Autodesk Inventor part; units mm, degrees
ref_plane "end_2_XY" through (22.3, 10.5, 6.25) normal (0, 1, 0) x (1, 0, 0)
ref_plane "end_2_YZ" through (22.3, 10.5, 6.25) normal (1, 0, 0) x (0, 0, -1)
ref_plane "end_2_ZX" through (22.3, 10.5, 6.25) normal (0, 0, -1) x (0, 1, 0)
sketch "Sketch_77" plane through (0, 0, 0) normal (0, 0, 1) x (1, 0, 0)
  line L0 (0, 7.9) -> (0, -7.9)
  line L1 (0, -7.9) -> (16, -7.9)
  line L2 (16, -7.9) -> (16, 7.9)
  line L3 (16, 7.9) -> (0, 7.9)
  circle A0 centre (12, 0) radius 1.5
  circle A1 centre (4, 0) radius 1.5
extrude "Extrusion1" add sketch "Sketch_77" along normal blind 2
sketch "Sketch_78" plane through (0, 7.9, 0) normal (0, 1, 0) x (1, 0, 0)
  arc A0 (0, -4.5344) -> (0.6773, -5.4809) centre (1, -4.5344) ccw
  line L0 (0.6773, -5.4809) -> (20.283, -12.1656)
  arc A1 (20.283, -12.1656) -> (22.3, 0) centre (22.3, -6.25) ccw
  line L1 (22.3, 0) -> (0, 0)
  line L2 (0, 0) -> (0, -4.5344)
extrude "Extrusion2" add sketch "Sketch_78" along normal blind 1.85
sketch "Sketch_79" plane through (0, -7.9, 0) normal (0, 1, 0) x (1, 0, 0)
  arc A0 (0, -4.5344) -> (0.6773, -5.4809) centre (1, -4.5344) ccw
  line L0 (0.6773, -5.4809) -> (20.283, -12.1656)
  arc A1 (20.283, -12.1656) -> (22.3, 0) centre (22.3, -6.25) ccw
  line L1 (22.3, 0) -> (0, 0)
  line L2 (0, 0) -> (0, -4.5344)
extrude "Extrusion3" add sketch "Sketch_79" against normal blind 1.85
sketch "Sketch_80" plane through (0, 9.6, 0) normal (0, 1, 0) x (1, 0, 0)
  circle A0 centre (22.3, -6.25) radius 3
extrude "Extrusion4" add sketch "Sketch_80" along normal blind 1.4
sketch "Sketch_81" plane through (0, -9.6, 0) normal (0, 1, 0) x (1, 0, 0)
  circle A0 centre (22.3, -6.25) radius 3
extrude "Extrusion5" add sketch "Sketch_81" along normal mid plane 2.8
sketch "Sketch_82" plane through (0, 9.6, 0) normal (0, 1, 0) x (1, 0, 0)
  arc A0 (0, -4.5344) -> (0.6773, -5.4809) centre (1, -4.5344) ccw
  line L0 (0.6773, -5.4809) -> (15.3, -10.4666)
  line L1 (15.3, -10.4666) -> (15.3, 0)
  line L2 (15.3, 0) -> (0, 0)
  line L3 (0, 0) -> (0, -4.5344)
extrude "Extrusion6" add sketch "Sketch_82" along normal blind 1.4
sketch "Sketch_83" plane through (0, -9.6, 0) normal (0, 1, 0) x (1, 0, 0)
  arc A0 (0, -4.5344) -> (0.6773, -5.4809) centre (1, -4.5344) ccw
  line L0 (0.6773, -5.4809) -> (15.3, -10.4666)
  line L1 (15.3, -10.4666) -> (15.3, 0)
  line L2 (15.3, 0) -> (0, 0)
  line L3 (0, 0) -> (0, -4.5344)
extrude "Extrusion7" add sketch "Sketch_83" along normal mid plane 2.8
ref_plane "end_2_XY" through (22.3, 10.5, 6.25) normal (0, 1, 0) x (1, 0, 0)
ref_plane "end_2_YZ" through (22.3, 10.5, 6.25) normal (1, 0, 0) x (0, 0, -1)
ref_plane "end_2_ZX" through (22.3, 10.5, 6.25) normal (0, 0, -1) x (0, 1, 0)
ref_plane "end_move_XY" through (22.3, -11.5, 6.25) normal (0, -1, 0) x (1, 0, 0)
ref_plane "end_move_YZ" through (22.3, -11.5, 6.25) normal (1, 0, 0) x (0, 0, 1)
ref_plane "end_move_ZX" through (22.3, -11.5, 6.25) normal (0, 0, 1) x (0, -1, 0)
ref_plane "to_dummy_XY" through (0, 0, 0) normal (0, 0, 1) x (1, 0, 0)
ref_plane "to_dummy_YZ" through (0, 0, 0) normal (1, 0, 0) x (0, 1, 0)
ref_plane "to_dummy_ZX" through (0, 0, 0) normal (0, 1, 0) x (0, 0, 1)
properties part number "045-16-2_se08f"
The listing builds one solid part. Answer for the finished solid, in the listing's coordinates (mm). A direction names the side the tool comes from. Coordinates: 2 decimals unless noted, no trailing zeros. Loops run counter-clockwise (first coordinate to the right, second up) from the corner with the lowest first, then second, coordinate; pieces in that order, holes last. Notation, with made-up numbers: (6, 31) - (63, 31) arc R31 ccw to (63, 68) - close; hole circle Ø4 at (86.25, -14.75). An arc over 180 degrees is marked (long way). Write item = value, one per line.
1) Section D-D (z = 6.25) is taken. Determine the outline of the cut face in (x, y), plus the area to 3 significant figures.
Responses:
outline = (2.93, -11) - (15.3, -11) - (15.3, -9.75) - (19.3, -9.75) - (19.3, -11) - (25.3, -11) - (25.3, -9.75) - (28.55, -9.75) - (28.55, -7.9) - (2.93, -7.9) - close; (2.93, 7.9) - (28.55, 7.9) - (28.55, 9.75) - (25.3, 9.75) - (25.3, 11) - (19.3, 11) - (19.3, 9.75) - (15.3, 9.75) - (15.3, 11) - (2.93, 11) - close
area = 141 mm^2
2) Find the intervals of material crossed by line 1 along Y through (x, z) = (12, 1.4); line 2 along Y through (x, z) = (4, 2.75); line 3 along Z through (x, y) = (4.75, -3.75), in increasing order.
Responses:
line_1 = -11 to -1.5, 1.5 to 11
line_2 = -11 to -7.9, 7.9 to 11
line_3 = 0 to 2
3) Section B-B (z = 2.5) is taken. Determine the outline of the cut face in (x, y).
Responses:
outline = (0, -11) - (15.3, -11) - (15.3, -9.75) - (27.3, -9.75) - (27.3, -7.9) - (0, -7.9) - close; (0, 7.9) - (27.3, 7.9) - (27.3, 9.75) - (15.3, 9.75) - (15.3, 11) - (0, 11) - close
4) Section C-C (x = 4) is taken. Determine the outline of the cut face in (y, z), plus the area to 3 significant figures.
Responses:
outline = (-11, 0) - (-1.5, 0) - (-1.5, 2) - (-7.9, 2) - (-7.9, 6.61) - (-11, 6.61) - close; (1.5, 0) - (11, 0) - (11, 6.61) - (7.9, 6.61) - (7.9, 2) - (1.5, 2) - close
area = 66.6 mm^2
5) Section A-A (y = 0) is taken. Determine the outline of the cut face in (x, z).
Responses:
outline = (0, 0) - (2.5, 0) - (2.5, 2) - (0, 2) - close; (5.5, 0) - (10.5, 0) - (10.5, 2) - (5.5, 2) - close; (13.5, 0) - (16, 0) - (16, 2) - (13.5, 2) - close
6) Which of the six approach directions +Z, -Z, +X, -X, +Y, -Y give full straight-line access (tool end or side, diameter ignored) to faces 1 (the face through (19, -9.75, 6)), 2 (the face through (16, 0, 1)), 3 (the face through (17, 7.9, 6))?
Responses:
face_1 = -Y
face_2 = +Z, -Z, +X
face_3 = +Z, +X
7) Determine the mould class of faces 4 (the face through (8, 11, 4)), 5 (the face through (10.5, -0.07, 0.99)), 6 (the face through (28.44, -8.81, 7.42)) for opening direction Y: pulls with the +Y half, pulls with the -Y half, needs draft (parallel to the pull), parting line crosses it, or undercut.
Responses:
face_4 = pulls with the +Y half
face_5 = undercut
face_6 = needs draft
8) Each of these flat-tipped pins is pushed along its axis until it touches: P1, Ø2.5, axis at x = 4, y = 0, coming from the +Z side; P2, Ø4, axis at x = 19, z = 4.5, coming from the +Y side; P3, Ø1, axis at y = -10.5, z = 7.5, coming from the +X side; P4, Ø6, axis at x = 4, y = -4, coming from the +Z side. Where does it stop, or does it pass through?
Responses:
P1 = through
P2 = 11
P3 = 25.2
P4 = 2
